Read the model definition and answer for the solid it produces. Units are mm, in the model's axes. Face numbers are marked on the shaded views. A direction names the side the tool comes from. Coordinates: 2 decimals unless noted, no trailing zeros. Order: outer loops, then holes, each group sorted by start corner. A loop starts at its lowest first (then second) coordinate and runs counter-clockwise, first axis right, second up. Notation, with made-up numbers: M -35,26.5 L -4,26.5 A18 ccw -4,46.5 Z; hole C 42.25,82 d11. An arc over 180 degrees is marked long. Use a Markdown table: item, result. Add a question column.
1) Find section B-B on y = 0. Write down the section's boundary in (x, z).
2) The mould has two halves that part along Y. Classify the marked faces 3, 4, 5 and 6: released by +Y, released by -Y, zero draft, split by the parting line, or undercut.
3) Find section A-A on z = 7.5. Count the separate pieces of the cut face and the enclosed holes in it, plus the area to 3 significant figures.
4) Find section C-C on z = -1. Write down the section's boundary in (x, y).
5) Find the intervals of material crossed by probe 1 along X at (y, z) = (0, 3); probe 2 along X at (y, z) = (0, 1.75); probe 3 along Y at (x, z) = (1, -1.75), in increasing order. Write a range as [from, to].
6) For the marked faces 1 and 2, determine the directions among +Z, -Z, +X, -X, +Y, -Y from which every point of the face is accessible in a straight line to the end or side of a thin tool.
7) Each of these flat-tipped pins is pushed along its axis until it touches: pin 1 Ø2 at (x, z) = (14, 6) entering from +Y; pin 2 Ø5 at (x, y) = (-1, -14.5) entering from -Z; pin 3 Ø10 at (x, y) = (-3.5, 2) entering from -Z; pin 4 Ø6 at (x, z) = (-8, 0.5) entering from -Y. Where does it stop, or does it pass through?
Autodesk Inventor part; units mm, degrees
ref_plane "Work Plane2" through (10, 17.3205, 3.1062) normal (0.5, 0.866, 0) x (-0.866, 0.5, 0)
ref_plane "XZ Plane" through (0, 0, 0) normal (0, 1, 0) x (-1, 0, 0)
ref_plane "XY Plane" through (0, 0, 0) normal (0, 0, 1) x (1, 0, 0)
sketch "Sketch1" plane through (0, 0, 0) normal (1, 0, 0) x (0, 1, 0)
  line L0 (0, 0) -> (0, -33.1818)
  line L1 (20, 10.1062) -> (20, -3.8938)
  line L2 (20, -3.8938) -> (12.6, -3.8938)
  line L3 (12.6, -3.8938) -> (12.6, -1.8938)
  line L4 (12.6, -1.8938) -> (3.5, -1.8938)
  line L5 (3.5, -1.8938) -> (3.5, 10.1062)
  line L6 (7.5, 10.1062) -> (7.5, 2.7186)
  line L7 (7.5, 2.7186) -> (12.6, 2.7186)
  line L8 (12.6, 2.7186) -> (12.6, 10.1062)
  line L9 (3.5, 10.1062) -> (7.5, 10.1062)
  line L10 (12.6, 10.1062) -> (20, 10.1062)
  dimension "d0" = 7
  dimension "d1" = 25.2
  dimension "d3" = 14
  dimension "d4" = 40
  dimension "d28" = 2
  dimension "d29" = 4
revolve "Revolution1" add sketch "Sketch1" angle 360 about axis through (0, 0, 0) along (0, 0, -1)
sketch "Sketch2" plane through (0, 0, 10.1062) normal (0, 0, 1) x (1, 0, 0)
  point P0 (0, 0)
  point P1 (0, 16)
  dimension "d6" = 16
hole "Hole1" at (0, 16, 10.1062) direction (0, 0, -1) diameter 5 end through all
pattern_circular "Circular Pattern1" count 6 over 360 about axis through (0, 0, 3.1062) along (0, 0, -1) of "Hole1"
ref_plane "Work Plane2" through (10, 17.3205, 3.1062) normal (0.5, 0.866, 0) x (-0.866, 0.5, 0)
ref_plane "Work Plane1" through (0, 0, 0) normal (0.5, 0.866, 0) x (0, 0, 1)
sketch "Sketch3" plane through (10, 17.3205, 3.1062) normal (0.5, 0.866, 0) x (-0.866, 0.5, 0)
  line L0 (-20, 7) -> (20, 7)
  line L1 (-20, -7) -> (20, -7)
  line L2 (0, 7) -> (0, -3.1062)
  point P0 (0, 1.9469)
hole "Hole2" at (10, 17.3205, 5.0531) direction (-0.5, -0.866, 0) diameter 6.647 depth 9.2 tip angle 118
chamfer "Chamfer1" distance 0.2 angle 45 4 edges at (0, -20, -3.8938) (0, -3.5, 10.1062) (0, -3.5, -1.8938) (0, -12.6, -1.8938)
properties part number "MirrorHeatsink" material "Copper"
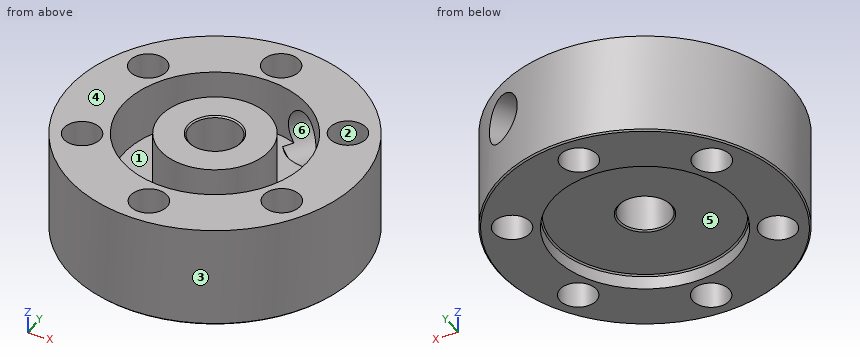
Check result:
| question | item | result |
|---|---|---|
| 1 | outline | M -20,-3.69 L -19.8,-3.89 L -12.6,-3.89 L -12.6,-2.09 L -12.4,-1.89 L -3.7,-1.89 L -3.5,-1.69 L -3.5,9.91 L -3.7,10.11 L -7.5,10.11 L -7.5,2.72 L -12.6,2.72 L -12.6,10.11 L -20,10.11 Z; M 3.5,-1.69 L 3.7,-1.89 L 12.4,-1.89 L 12.6,-2.09 L 12.6,-3.89 L 19.8,-3.89 L 20,-3.69 L 20,10.11 L 12.6,10.11 L 12.6,2.72 L 7.5,2.72 L 7.5,10.11 L 3.7,10.11 L 3.5,9.91 Z |
| 2 | face 3 | split by the parting line |
| 2 | face 4 | zero draft |
| 2 | face 5 | undercut |
| 2 | face 6 | undercut |
| 3 | separate pieces | 2 |
| 3 | enclosed holes | 7 |
| 3 | area | 745 mm2 |
| 4 | outline | C 0,0 d40; hole C -13.86,-8 d5; hole C -13.86,8 d5; hole C 0,0 d7; hole C 0,-16 d5; hole C 0,16 d5; hole C 13.86,-8 d5; hole C 13.86,8 d5 |
| 5 | probe 1 | x = [-20, -12.6], [-7.5, -3.5], [3.5, 7.5], [12.6, 20] |
| 5 | probe 2 | x = [-20, -3.5], [3.5, 20] |
| 5 | probe 3 | y = [-19.97, -18.29], [-13.71, -3.41], [3.41, 13.71], [18.29, 19.97] |
| 6 | face 1 | +Z |
| 6 | face 2 | +Z, -Z |
| 7 | pin 1 | stops at y = 15.2 |
| 7 | pin 2 | stops at z = -3.89 |
| 7 | pin 3 | stops at z = -1.89 |
| 7 | pin 4 | stops at y = -19.36 |
